Geometry check sheet. Reference: the model listing, model coordinates, mm. A direction names the side the tool comes from. Round coordinates to 2 decimals unless told otherwise and drop trailing zeros. Write each loop counter-clockwise with the first axis right and the second up, starting at its lowest first coordinate (ties: lowest second). Pieces come first, ordered by that corner, then holes.
from build123d import *

# Parameters (mm, degrees)
BOSS_EXTRUDE1_DEPTH = 8.382
CUT_EXTRUDE2_DEPTH  = 2.032
SKETCH4_R           = 3.3274
SKETCH4_R_2         = 1.27
CUT_EXTRUDE3_DEPTH  = 3.032
CUT_EXTRUDE4_DEPTH  = 2.4257


with BuildPart() as part:
    # Sketch1 → Boss-Extrude1 (new body, symmetric)
    with BuildSketch(Plane.XY):
        with BuildLine():
            Line((0, 0), (-25.4, 0))
            ThreePointArc((-25.4, 0), (-32.797029365, 17.124880227), (-15.258381189, 10.77087469))
            Line((-15.258381189, 10.77087469), (-14.732, 2.032))
            Line((-14.732, 2.032), (0, 2.032))
            Line((0, 2.032), (0, 0))
        make_face()
        with BuildLine():
            Line((-25.4, 3.81), (-18.660167236, 3.81))
            Line((-18.660167236, 3.81), (-19.079451597, 10.77087469))
            ThreePointArc((-19.079451597, 10.77087469), (-30.101146364, 14.428691001), (-25.4, 3.81))
        make_face(mode=Mode.SUBTRACT)
    extrude(amount=BOSS_EXTRUDE1_DEPTH, both=True)

    # Sketch3 → Cut-Extrude2 (cut)
    with BuildSketch(Plane(origin=(0, 2.032, 0), x_dir=(1, 0, 0), z_dir=(0, 1, 0))):
        with BuildLine():
            Line((0, -8.382), (0, 0))
            ThreePointArc((0, 0), (-0.55079832, -4.328930418), (-2.168093689, -8.382))
            Line((-2.168093689, -8.382), (0, -8.382))
        make_face()
        with BuildLine():
            Line((0, 0), (0, 8.382))
            Line((0, 8.382), (-2.168093689, 8.382))
            ThreePointArc((-2.168093689, 8.382), (-0.55079832, 4.328930418), (0, 0))
        make_face()
    extrude(amount=-CUT_EXTRUDE2_DEPTH, mode=Mode.SUBTRACT)

    # Sketch4 → Cut-Extrude3 (cut, through all)
    with BuildSketch(Plane(origin=(0, 2.032, 0), x_dir=(1, 0, 0), z_dir=(0, 1, 0))):
        with Locations((-7.366, 0)):
            Circle(SKETCH4_R)
        with Locations((-13.716, 0)):
            Circle(SKETCH4_R_2)
    extrude(amount=-CUT_EXTRUDE3_DEPTH, mode=Mode.SUBTRACT)

    # Sketch5 → Cut-Extrude4 (cut, symmetric)
    with BuildSketch(Plane.XY):
        with BuildLine():
            Line((-25.4, 0), (-18.430674034, 0))
            Line((-18.430674034, 0), (-18.514821541, 1.397))
            Line((-18.514821541, 1.397), (-25.4, 1.397))
            ThreePointArc((-25.4, 1.397), (-31.779937827, 16.167209196), (-16.652853775, 10.68687942))
            Line((-16.652853775, 10.68687942), (-16.131531994, 2.032))
            Line((-16.131531994, 2.032), (-14.732, 2.032))
            Line((-14.732, 2.032), (-15.258381189, 10.77087469))
            ThreePointArc((-15.258381189, 10.77087469), (-32.797029365, 17.124880227), (-25.4, 0))
        make_face()
    extrude(amount=CUT_EXTRUDE4_DEPTH, both=True, mode=Mode.SUBTRACT)


solid = part.part
1. Scan lines: line 1 along Z through (x, y) = (-34, 8); line 2 along Y through (x, z) = (-25.4, 4.5); line 3 along Y through (x, z) = (-7, -3.75). Record each from-to range of solid material in increasing order.
2. Section check B-B (z = -6). Record the cut outline in (x, y).
3. Depth check by flat-ended pin: pin 1 Ø4 at (y, z) = (17, 2.5) entering from -X; pin 2 Ø2.5 at (x, z) = (-22, -0.5) entering from -Y; pin 3 Ø5 at (y, z) = (10.5, -2) entering from +X. Enter the tip coordinate at first touch or a pass-through.
4. Access from +Z, -Z, +X, -X, +Y, -Y to the whole of each face (thin tool, end or side, straight path). Record for faces 1 (the face through (-31.97, 15.96, 0.03)), 2 (the face through (-22, 3.81, 0)), 3 (the face through (-16.396, 6.42, 0.034)), 4 (the face through (-15, 6.5, 5.4)).
5. Release check for a two-part mould opening along X. For faces 5 (the face through (-34, 7, 2.426)), 6 (the face through (-18.867, 7.242, 0.117)), 7 (the face through (-18.472, 0.689, 0.034)) record: +X half, -X half, draft (parallel to the pull), parting line (faces both ways), or undercut.
6. Section check D-D (z = 5). Record the cut outline in (x, y).
7. Section check C-C (x = -9). Record the cut outline in (y, z), plus the area to 3 significant figures.
8. Section check A-A (y = 6.5). Record the cut outline in (x, z), plus the area to 3 significant figures.
Results below:
1. line 1: z = -8.38 to -2.43, 2.43 to 8.38
1. line 2: y = 0 to 3.81, 16.51 to 20.32
1. line 3: y = 0 to 2.03
2. outline: (-25.4, 0) - (-1.07, 0) - (-1.07, 2.03) - (-14.73, 2.03) - (-15.26, 10.77) arc R10.16 ccw (long way) to start; hole (-25.4, 3.81) - (-18.66, 3.81) - (-19.08, 10.77) arc R6.35 ccw (long way) to start
3. pin 1: stops at x = -34.33
3. pin 2: stops at y = 1.4
3. pin 3: stops at x = -15.09
4. face 1: none
4. face 2: +Z, -Z
4. face 3: +X, +Y
4. face 4: +Z, -Z, +X, +Y
5. face 5: draft
5. face 6: undercut
5. face 7: -X half
6. outline: (-25.4, 0) - (-0.74, 0) - (-0.74, 2.03) - (-14.73, 2.03) - (-15.26, 10.77) arc R10.16 ccw (long way) to start; hole (-25.4, 3.81) - (-18.66, 3.81) - (-19.08, 10.77) arc R6.35 ccw (long way) to start
7. outline: (0, -8.38) - (2.03, -8.38) - (2.03, -2.9) - (0, -2.9) - close; (0, 2.9) - (2.03, 2.9) - (2.03, 8.38) - (0, 8.38) - close
7. area: 22.3 mm2
8. outline: (-34.88, -8.38) - (-30.59, -8.38) - (-30.59, 8.38) - (-34.88, 8.38) - (-34.88, 2.43) - (-33.36, 2.43) - (-33.36, -2.43) - (-34.88, -2.43) - close; (-18.82, -8.38) - (-15, -8.38) - (-15, -2.43) - (-16.4, -2.43) - (-16.4, 2.43) - (-15, 2.43) - (-15, 8.38) - (-18.82, 8.38) - close
8. area: 122 mm2
